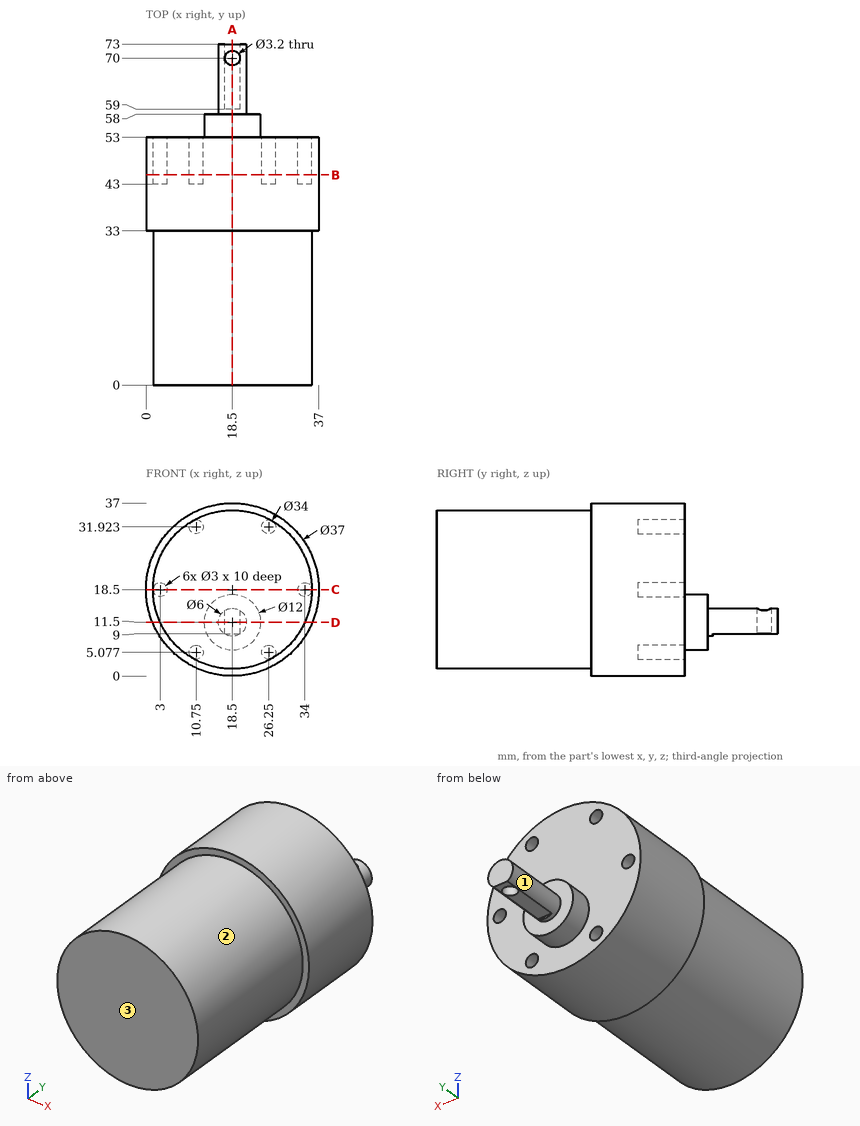
Source: three-view drawing plus pictorial views. Frame: mm from the lowest corner of the part. A direction names the side the tool comes from. Give positions to 0.01 mm unless a question says otherwise; leave off trailing zeros. Loops run counter-clockwise (first coordinate to the right, second up) from the corner with the lowest first, then second, coordinate; pieces in that order, holes last. Notation, with made-up numbers: (39, 63.25) -> (66, 63.25) arc R6 ccw to (66, 71.25) -> close; hole circle Ø11 at (30.5, -6). An arc over 180 degrees is marked (long way). Use a Markdown table: item, result. Add a question column.
(1) Section query B-B (y = 45). Output: boundary loops of the cut face in (x, z), then the cut area to 3 significant figures.
(2) First-contact query: pin 1 Ø1.5 at (y, z) = (12, 13.5) entering from -X; pin 2 Ø10 at (x, y) = (16.5, 19) entering from +Z; pin 3 Ø3.5 at (x, z) = (34, 18.5) entering from +Y. Flat tips, straight axial feed; report the tip coordinate or a pass-through.
(3) Section query C-C (z = 18.5). Output: boundary loops of the cut face in (x, y).
(4) Section query A-A (x = 18.5). Output: boundary loops of the cut face in (y, z), then the cut area to 3 significant figures.
(5) Ray query, line 1 (X direction, y = 49.5, z = 33) (1 decimal); line 2 (Y direction, x = 21.5, z = 14); line 3 (Y direction, x = 13, z = 17.5). Return the intervals inside material, ascending.
(6) Access query for the marked faces 1, 2 and 3. Directions: +Z, -Z, +X, -X, +Y, -Y. A direction counts if a zero-diameter tool reaches every point of the face in a straight line with its end or side. Return the directions, or none.
(7) Section query D-D (z = 11.5). Output: boundary loops of the cut face in (x, y) (1 decimal).
Checked values:
| question | item | result |
|---|---|---|
| 1 | outline | circle Ø37 at (18.5, 18.5); hole circle Ø3 at (3, 18.5); hole circle Ø3 at (10.75, 5.08); hole circle Ø3 at (10.75, 31.92); hole circle Ø3 at (26.25, 5.08); hole circle Ø3 at (26.25, 31.92); hole circle Ø3 at (34, 18.5) |
| 1 | area | 1,030 mm^2 |
| 2 | pin 1 | x = 2.04 |
| 2 | pin 2 | z = 35.5 |
| 2 | pin 3 | y = 53 |
| 3 | outline | (0, 33) -> (1.5, 33) -> (1.5, 0) -> (35.5, 0) -> (35.5, 33) -> (37, 33) -> (37, 53) -> (35.5, 53) -> (35.5, 43) -> (32.5, 43) -> (32.5, 53) -> (4.5, 53) -> (4.5, 43) -> (1.5, 43) -> (1.5, 53) -> (0, 53) -> close |
| 4 | outline | (0, 1.5) -> (33, 1.5) -> (33, 0) -> (53, 0) -> (53, 5.5) -> (58, 5.5) -> (58, 8.5) -> (59, 8.5) -> (59, 9) -> (68.4, 9) -> (68.4, 14.5) -> (58, 14.5) -> (58, 17.5) -> (53, 17.5) -> (53, 37) -> (33, 37) -> (33, 35.5) -> (0, 35.5) -> close; (71.6, 9) -> (73, 9) -> (73, 14.5) -> (71.6, 14.5) -> close |
| 4 | area | 1,990 mm^2 |
| 5 | line 1 | 7 to 9.7, 11.8 to 25.2, 27.3 to 30 |
| 5 | line 2 | 0 to 58 |
| 5 | line 3 | 0 to 53 |
| 6 | face 1 | +Y |
| 6 | face 2 | -Y |
| 6 | face 3 | +Z, -Z, +X, -X, -Y |
| 7 | outline | (1.4, 33) -> (3, 33) -> (3, 0) -> (34, 0) -> (34, 33) -> (35.6, 33) -> (35.6, 53) -> (24.5, 53) -> (24.5, 58) -> (21.5, 58) -> (21.5, 73) -> (15.5, 73) -> (15.5, 58) -> (12.5, 58) -> (12.5, 53) -> (1.4, 53) -> close; hole circle Ø3.2 at (18.5, 70) |
